Model file for the job. Use its own axes, mm. Face numbers are marked on the shaded views. A direction names the side the tool comes from. Coordinates: 2 decimals unless noted, no trailing zeros. Order: outer loops, then holes, each group sorted by start corner. A loop starts at its lowest first (then second) coordinate and runs counter-clockwise, first axis right, second up.
from build123d import *

# Parameters (mm, degrees)
F0_R            = 10
F1_DEPTH        = 3
F2_R            = 6
F3_DEPTH        = 3
F4_R            = 10
F4_R_2          = 6
F5_DEPTH        = 3
F6_SIZE         = 1
F8_D            = 2
F8_DEPTH        = 27
F8_CBORE_D      = 6
F8_CBORE_DEPTH  = 1.2
F8_TIP          = 0.600860619
F10_D           = 2
F10_DEPTH       = 9
F10_CBORE_D     = 3
F10_CBORE_DEPTH = 1.2
F10_TIP         = 0.600860619


with BuildPart() as f1:
    # F0 (on Top) → F1 (new body)
    with BuildSketch(Plane.XY):
        Circle(F0_R)
    extrude(amount=F1_DEPTH)

    # F2 (on face) → F3 (join)
    with BuildSketch(Plane.XY):
        Circle(F2_R)
    extrude(amount=-F3_DEPTH)

    # F4 (on face) → F5 (join)
    with BuildSketch(Plane(origin=(0, 0, -3), x_dir=(1, 0, 0), z_dir=(0, 0, -1))):
        Circle(F4_R)
        Circle(F4_R_2, mode=Mode.SUBTRACT)
        Circle(F4_R_2)
    extrude(amount=F5_DEPTH)

    # F6
    f6_edges = [f1.edges().sort_by_distance(p)[0] for p in [
        (-6, 0, 0),
        (-10, 0, -3),
        (-10, 0, 0),
        (-6, 0, -3),
        (-10, 0, -6),
    ]]
    chamfer(f6_edges, length=F6_SIZE)

    # F8
    with Locations(Plane(origin=(0, 0, -6), x_dir=(1, 0, 0), z_dir=(0, 0, -1))):
        with Locations((0, 0)):
            CounterBoreHole(F8_D / 2, F8_CBORE_D / 2, F8_CBORE_DEPTH, depth=F8_DEPTH)
            with Locations((0, 0, -(F8_DEPTH + F8_TIP / 2))):  # 118° drill point
                Cone(0, F8_D / 2, F8_TIP, mode=Mode.SUBTRACT)

    # F10
    with Locations(Plane(origin=(0, 0, -6), x_dir=(1, 0, 0), z_dir=(0, 0, -1))):
        with Locations((-4.575991758, 2.8671064562)):
            CounterBoreHole(F10_D / 2, F10_CBORE_D / 2, F10_CBORE_DEPTH, depth=F10_DEPTH)
            with Locations((0, 0, -(F10_DEPTH + F10_TIP / 2))):  # 118° drill point
                Cone(0, F10_D / 2, F10_TIP, mode=Mode.SUBTRACT)


solid = f1.part
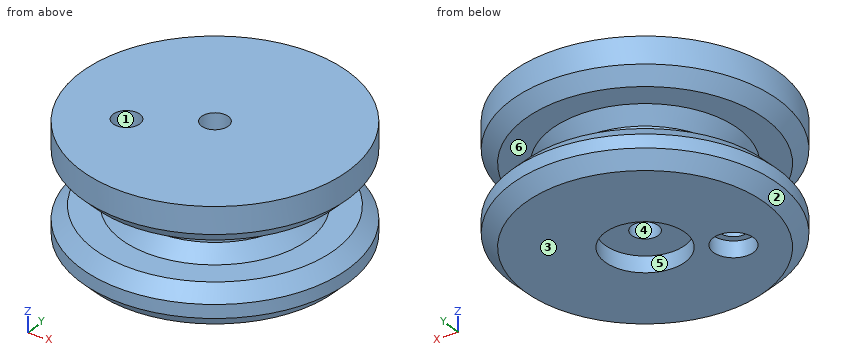
Q1. Mould opens along Y. For the marked faces 1, 2 and 3 say: pulls with the +Y half, pulls with the -Y half, needs draft (parallel to the pull), parting line crosses it, or undercut.
Established:
face 1: undercut
face 2: parting line crosses it
face 3: needs draft
Q2. Cut at D-D, the plane z = -1.5. List the corners of the cut face in (x, y), plus the area to 3 significant figures.
Established:
outline: (-5.48, -2.44) arc R1 cw (long way) to (-4.59, -3.87) arc R6 ccw (long way) to start; hole circle Ø2 at (0, 0)
area: 107 mm2
Q3. Which spindle directions (+Z, -Z, +X, -X, +Y, -Y) get a long thin tool onto all of the face, cutting with end or side? Do the marked faces 4, 5 and 6. Say none if no direction does.
Established:
face 4: +Z, -Z
face 5: -Z
face 6: none
Q4. Cut at C-C, the plane z = 2.25. List the corners of the cut face in (x, y).
Established:
outline: circle Ø20 at (0, 0); hole circle Ø2 at (-4.58, -2.87); hole circle Ø2 at (0, 0)
Q5. Probe line 1 (Z direction, x = 0.25, y = -8.5); line 2 (Y direction, x = 0, z = 1.5); line 3 (Z direction, x = 0.75, y = -1). List the from-to ranges inside material, lowest first.
Established:
line 1: z = -6 to -3, 0 to 3
line 2: y = -10 to -1, 1 to 10
line 3: z = -4.8 to 3
Q6. Drop flat-ended pins along their axis: P1, Ø2.5, axis at x = -5.5, y = -2.5, coming from the -Z side; P2, Ø3.5, axis at x = 0, y = 0, coming from the -Z side. Give the stop position or say it passes through.
Established:
P1: stops at z = -6
P2: stops at z = -4.8
